Could you check a few things on this model? Use its own coordinates, in mm. Face numbers are marked on the shaded views. A direction names the side the tool comes from. Coordinates: 2 decimals unless noted, no trailing zeros. Write each loop counter-clockwise with the first axis right and the second up, starting at its lowest first coordinate (ties: lowest second). Pieces come first, ordered by that corner, then holes. Notation, with made-up numbers: M -36.75,-0.5 L 17.25,-0.5 A11 cw 17.25,19.5 Z; hole C 81,62 d1. An arc over 180 degrees is marked long. Write item = value, one per line.
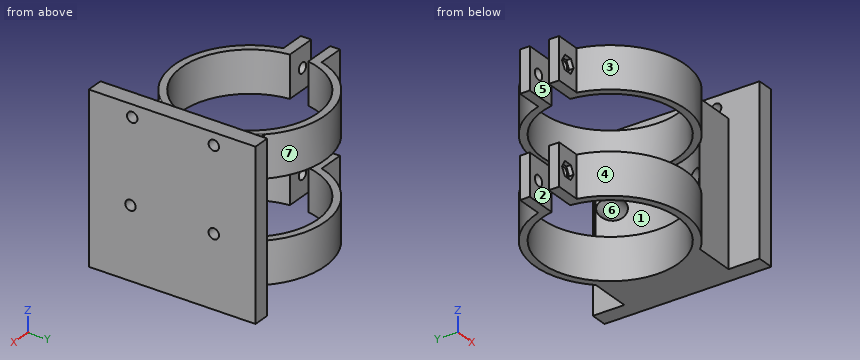
```python
from build123d import *

# Parameters (mm, degrees)
BOSS_EXTRU_2_DEPTH         = 20
BOSS_EXTRU_4_DEPTH         = 2.2401
BOSS_EXTRU_4_DEPTH_BACK    = 20
ESQUISSE3_R                = 2.5
BOSS_EXTRU_7_DEPTH         = 6.805036811
BOSS_EXTRU_7_DEPTH_BACK    = 0.2
ESQUISSE13_W               = 8
ESQUISSE13_H               = 80
BOSS_EXTRU_9_DEPTH         = 80
BOSS_EXTRU_11_DEPTH        = 40
BOSS_EXTRU_11_DEPTH_BACK   = 3.5598
ESQUISSE16_R               = 2.5
BOSS_EXTRU_11_2_DEPTH      = 40
BOSS_EXTRU_11_2_DEPTH_BACK = 3.5598
BOSS_EXTRU_11_3_DEPTH      = 40
BOSS_EXTRU_11_3_DEPTH_BACK = 3.5598
BOSS_EXTRU_11_4_DEPTH      = 40
BOSS_EXTRU_11_4_DEPTH_BACK = 3.5598
BOSS_EXTRU_12_DEPTH        = 68
ESQUISSE19_R               = 5.214324904
BOSS_EXTRU_15_DEPTH        = 21.55
ESQUISSE19_R_2             = 5
BOSS_EXTRU_15_2_DEPTH      = 21.55


with BuildPart() as part:
    # Esquisse1 → Boss.-Extru.2 (new body)
    with BuildSketch(Plane.XY):
        with BuildLine():
            Line((-71.273833315, 9.654910047), (-56.622475708, 9.654910047))
            ThreePointArc((-56.622475708, 9.654910047), (8.178325953, 11.885050452), (-56.29470269, 18.765893404))
            Line((-56.29470269, 18.765893404), (-71.29470269, 18.765893404))
            Line((-71.29470269, 18.765893404), (-71.29470269, 23.440192667))
            Line((-71.29470269, 23.440192667), (-58.769730896, 23.440192667))
            ThreePointArc((-58.769730896, 23.440192667), (11.684606541, 12.02375525), (-59.307286147, 4.654910047))
            Line((-59.307286147, 4.654910047), (-71.273833315, 4.654910047))
            Line((-71.273833315, 4.654910047), (-71.273833315, 9.654910047))
        make_face()
    extrude(amount=BOSS_EXTRU_2_DEPTH)


with BuildPart() as body_2:
    # Esquisse3 → Boss.-Extru.4 (new, two sides: drawn at the far end of the back side and taken through both)
    with BuildSketch(Plane(origin=(11.50882306, 4.654910047, -20.756809104), x_dir=(-1, 0, 0), z_dir=(0, -1, 0)).offset(-BOSS_EXTRU_4_DEPTH_BACK)):
        with Locations(Location((76.783055813, -30.756809104, 0), (0, 0, 90))):
            Circle(ESQUISSE3_R)
    extrude(amount=BOSS_EXTRU_4_DEPTH + BOSS_EXTRU_4_DEPTH_BACK)


with BuildPart() as body_3:
    # Esquisse8 → Boss.-Extru.7 (new, two sides: drawn at the far end of the back side and taken through both)
    with BuildSketch(Plane(origin=(38.166060495, 0, 0), x_dir=(1, 0, 0), z_dir=(0, 1, 0)).offset(-BOSS_EXTRU_7_DEPTH_BACK)):
        Polygon((-101.475254656, -13.421592672), (-99.52284996, -9.930444451), (-101.570070661, -6.494038275), (-105.569696057, -6.548780321), (-107.522100752, -10.039928543), (-105.474880052, -13.476334718), align=None)
    extrude(amount=BOSS_EXTRU_7_DEPTH + BOSS_EXTRU_7_DEPTH_BACK)


with BuildPart() as part_1:
    add(part.part)

    # Combiner2: cut body 2, body 3
    add(body_2.part, mode=Mode.SUBTRACT)
    add(body_3.part, mode=Mode.SUBTRACT)


with BuildPart() as body_2_2:
    # Corps-Déplacer/Copier2: copy of part
    add(part_1.part.moved(Location((0, 0, 72.964959744))))


with BuildPart() as body_3_2:
    # Esquisse13 → Boss.-Extru.9 (new body)
    with BuildSketch(Plane.XY):
        with Locations((26.041295444, 19.15878473)):
            Rectangle(ESQUISSE13_W, ESQUISSE13_H)
    extrude(amount=BOSS_EXTRU_9_DEPTH)


with BuildPart() as body_2_2_1:
    # Corps-Déplacer/Copier3: moved
    add(body_2_2.part.moved(Location((0, 0, -25))))


with BuildPart() as body_4:
    # Esquisse16 → Boss.-Extru.11 (new, two sides: drawn at the far end of the back side and taken through both)
    with BuildSketch(Plane(origin=(0, 0, 0), x_dir=(0, 0, -1), z_dir=(1, 0, 0)).offset(-BOSS_EXTRU_11_DEPTH_BACK)):
        with Locations((-34.262679566, 39.15878473)):
            Circle(ESQUISSE16_R)
    extrude(amount=BOSS_EXTRU_11_DEPTH + BOSS_EXTRU_11_DEPTH_BACK)


with BuildPart() as body_5:
    # Esquisse16 → Boss.-Extru.11 2 (new, two sides: drawn at the far end of the back side and taken through both)
    with BuildSketch(Plane(origin=(0, 0, 0), x_dir=(0, 0, -1), z_dir=(1, 0, 0)).offset(-BOSS_EXTRU_11_2_DEPTH_BACK)):
        with Locations((-34.195620058, -0.841159058)):
            Circle(ESQUISSE16_R)
    extrude(amount=BOSS_EXTRU_11_2_DEPTH + BOSS_EXTRU_11_2_DEPTH_BACK)


with BuildPart() as body_6:
    # Esquisse16 → Boss.-Extru.11 3 (new, two sides: drawn at the far end of the back side and taken through both)
    with BuildSketch(Plane(origin=(0, 0, 0), x_dir=(0, 0, -1), z_dir=(1, 0, 0)).offset(-BOSS_EXTRU_11_3_DEPTH_BACK)):
        with Locations((-74.176398553, 0)):
            Circle(ESQUISSE16_R)
    extrude(amount=BOSS_EXTRU_11_3_DEPTH + BOSS_EXTRU_11_3_DEPTH_BACK)


with BuildPart() as body_7:
    # Esquisse16 → Boss.-Extru.11 4 (new, two sides: drawn at the far end of the back side and taken through both)
    with BuildSketch(Plane(origin=(0, 0, 0), x_dir=(0, 0, -1), z_dir=(1, 0, 0)).offset(-BOSS_EXTRU_11_4_DEPTH_BACK)):
        with Locations((-74.176398553, 39.15878473)):
            Circle(ESQUISSE16_R)
    extrude(amount=BOSS_EXTRU_11_4_DEPTH + BOSS_EXTRU_11_4_DEPTH_BACK)


with BuildPart() as body_3_2_1:
    add(body_3_2.part)

    # Combiner3: cut body 7, body 4, body 6, body 5
    add(body_7.part, mode=Mode.SUBTRACT)
    add(body_4.part, mode=Mode.SUBTRACT)
    add(body_6.part, mode=Mode.SUBTRACT)
    add(body_5.part, mode=Mode.SUBTRACT)


with BuildPart() as part_2:
    add(part_1.part)

    add(body_2_2_1.part)  # Boss.-Extru.12 merges body 2 2
    # Esquisse17 → Boss.-Extru.12 (add)
    with BuildSketch(Plane.XY):
        with BuildLine():
            Line((21.259619395, 38.041540738), (1.098292972, 38.041540738))
            Line((1.098292972, 38.041540738), (1.098292972, 37.989779899))
            ThreePointArc((1.098292972, 37.989779899), (11.250408812, 13.048189822), (1.259619395, -11.958459262))
            Line((1.259619395, -11.958459262), (21.259619395, -11.958459262))
            Line((21.259619395, -11.958459262), (21.259619395, 38.041540738))
        make_face()
    extrude(amount=BOSS_EXTRU_12_DEPTH)


with BuildPart() as body_3_2_2:
    # Corps-Déplacer/Copier4: moved
    add(body_3_2_1.part.moved(Location((0, -10, 0))))


with BuildPart() as body_3_2_3:
    # Corps-Déplacer/Copier5: moved
    add(body_3_2_2.part.moved(Location((0, 5, 0))))


with BuildPart() as body_3_2_4:
    # Corps-Déplacer/Copier6: moved
    add(body_3_2_3.part.moved(Location((0, -1, 0))))


with BuildPart() as body_3_2_5:
    # Corps-Déplacer/Copier7: moved
    add(body_3_2_4.part.moved(Location((57.599184588, 0, 0))))


with BuildPart() as part_3:
    # Corps-Déplacer/Copier8: moved
    add(part_2.part.moved(Location((-92, 0, 0))))


with BuildPart() as body_3_3:
    # Esquisse19 → Boss.-Extru.15 (new body)
    with BuildSketch(Plane(origin=(0, 0, 0), x_dir=(0, 0, -1), z_dir=(1, 0, 0))):
        with Locations((-34.195620058, 32.532899017)):
            Circle(ESQUISSE19_R)
    extrude(amount=BOSS_EXTRU_15_DEPTH)


with BuildPart() as body_4_2:
    # Esquisse19 → Boss.-Extru.15 2 (new body)
    with BuildSketch(Plane(origin=(0, 0, 0), x_dir=(0, 0, -1), z_dir=(1, 0, 0))):
        with Locations((-34.195620058, -6.841159058)):
            Circle(ESQUISSE19_R_2)
    extrude(amount=BOSS_EXTRU_15_2_DEPTH)


with BuildPart() as part_4:
    # Corps-Déplacer/Copier9: moved
    add(part_3.part.moved(Location((91.524740037, 0, 0))))

    # Combiner6: cut body 3 3, body 4 2
    add(body_3_3.part, mode=Mode.SUBTRACT)
    add(body_4_2.part, mode=Mode.SUBTRACT)


with BuildPart() as body_3_2_6:
    # Corps-Déplacer/Copier12: moved
    add(body_3_2_5.part.moved(Location((-59, 0, 0))))

    # Combiner7: union part
    add(part_4.part)


solid = body_3_2_6.part
```
Item 1: I'm going to push flat-ended pins straight in: P1, Ø10, axis at x = 12, z = 35.5, coming from the -Y side; P2, Ø8, axis at y = -6.84, z = 34.2, coming from the -X side; P3, Ø12, axis at x = 2.5, z = 55, coming from the -Y side. Where does each tip first touch, or does it pass through?
Numbers:
P1 = -11.96
P2 = 20.64
P3 = -15.99
Item 2: If we mould it in two halves opening along X, with no side actions, what happens to the marked faces 1, 2, 3 and 4? For each: pulls with the +X half, pulls with the -X half, needs draft (parallel to the pull), parting line crosses it, or undercut.
Numbers:
face_1 = pulls with the -X half
face_2 = needs draft
face_3 = undercut
face_4 = undercut
Item 3: Imagine slicing it at A-A (x = -9). Write out the boundary of the cut face in (y, z).
Numbers:
outline = M -19.31,0 L -15.36,0 L -15.36,20 L -19.31,20 Z; M -19.31,47.96 L -15.36,47.96 L -15.36,67.96 L -19.31,67.96 Z; M 41.47,0 L 45.41,0 L 45.41,20 L 41.47,20 Z; M 41.47,47.96 L 45.41,47.96 L 45.41,67.96 L 41.47,67.96 Z
Item 4: Imagine slicing it at B-B (z = 23). Write out the boundary of the cut face in (x, y).
Numbers:
outline = M 0.62,37.99 A36 cw 0.78,-11.96 L 20.64,-11.96 L 20.64,-26.84 L 28.64,-26.84 L 28.64,53.16 L 20.64,53.16 L 20.64,38.04 L 0.62,38.04 Z
Item 5: Imagine slicing it at D-D (y = 40.5). Write out the boundary of the cut face in (x, z).
Numbers:
outline = M -48.07,0 L -42.18,0 L -42.18,20 L -48.07,20 Z; M -48.07,47.96 L -42.18,47.96 L -42.18,67.96 L -48.07,67.96 Z; M -7.37,0 L -1.48,0 L -1.48,20 L -7.37,20 Z; M -7.37,47.96 L -1.48,47.96 L -1.48,67.96 L -7.37,67.96 Z; M 20.64,0 L 28.64,0 L 28.64,80 L 20.64,80 Z
Item 6: If I drill on line 1 along X through (y, z) = (20, 10); line 2 along Y through (x, z) = (-61, 9); line 3 along Z through (x, y) = (-57, 1.5), over which ranges is the centre line in solid material (lowest first)?
Numbers:
line_1 = -71.77 to -68.25, -63.25 to -56.52, 6.97 to 28.64
line_2 = 4.65 to 9.65, 18.77 to 23.44
line_3 = 0 to 20, 47.96 to 67.96
Item 7: For the marked faces 5, 6 and 7, which set-ups out of +Z, -Z, +X, -X, +Y, -Y let a thin tool reach every point of the face, with its end or its side?
Numbers:
face_5 = +Z, -Z, -X
face_6 = -X
face_7 = +Z, -Z, +Y
Item 8: Imagine slicing it at C-C (y = 21.5). State how many separate pieces and enclosed holes the cut face has, and give its area (3 significant figures).
Numbers:
separate_pieces = 3
enclosed_holes = 2
area = 2,090 mm²
